Autodesk Fusion 360 part; units mm, degrees
sketch "Sketch1" plane through (0, 0, 0) normal (0, 1, 0) x (1, 0, 0)
  circle A0 centre (0, 0) radius 10.5
  circle A1 centre (0, -0.5) radius 9.25
  line L0 (8, 12) -> (0, 0)
  line L1 (0, 0) -> (-8, 12)
  line L2 (-12, -8) -> (0, 0)
  line L3 (0, 0) -> (12, -8)
  circle A2 centre (0, 0) radius 8
  line L4 (6, 8) -> (6, -7)
  line L5 (-6, 8) -> (-6, -7)
  point P0 (0, -0.5)
  dimension "d1" = 21
  dimension "d2" = 0.5
  dimension "d3" = 18.5
  dimension "d4" = 16
extrude "Extrude1" add sketch "Sketch1" along normal blind 9 contours A0 A1 L0 L3 | A0 A1 L2 L3 | A0 A1 L1 L2 | A1 L0 A2 L4 | A1 L3 A2 L4 | A1 L2 L3 A2 | A1 L1 A2 L5 | A1 L2 A2 L5
extrude "Extrude2" add sketch "Sketch1" against normal blind 20 contours A0 A1 L0 L3 | A0 A1 L1 L2
extrude "Extrude3" add sketch "Sketch1" along normal blind 2 contours L3 A2 L4 | L3 A2 L4 | L2 A2 L5 | L2 A2 L5
chamfer "Chamfer1" distance 1.5 angle 45 1 edges at (8, 2, 0)
chamfer "Chamfer1" distance 1.5 angle 45 1 edges at (-8, 2, 0)
mirror "Mirror1" about plane through (0, 9, 0) normal (0, 1, 0) of bodies 1 merged
Here's how the part is built. I have some questions about the finished solid (model axes, mm). A direction names the side the tool comes from. Coordinates: 2 decimals unless noted, no trailing zeros. Loops run counter-clockwise (first coordinate to the right, second up) from the corner with the lowest first, then second, coordinate; pieces in that order, holes last.
1. Imagine slicing it at B-B, the plane z = 0. Please give me the cut outline in (x, y).
2. Imagine slicing it at A-A, the plane y = 25. Please give me the cut outline in (x, z), and give its area (3 significant figures).
3. Imagine slicing it at C-C, the plane x = -2.75. Please give me the cut outline in (y, z), and give its area (3 significant figures).
4. I need wall thicknesses on L1, parallel to Y at x = -2.5, z = 9; L2, parallel to X at y = 10.5, z = 0; L3, parallel to X at y = -6.5, z = -7. Which ranges of each line are inside material? Lowest first, please.
5. For faces 1 (the flat face through (-4, 18, 7.4)), 2 (the conical face through (-7.1, 15.4, 0.1)), 3 (the cylindrical face through (9.02, -9.86, -1.55)), which set-ups out of +Z, -Z, +X, -X, +Y, -Y let a thin tool reach every point of the face, with its end or its side?
6. If we mould it in two halves opening along X, with no side actions, what happens to faces 4 (the flat face through (9, -20, -3)), 5 (the cylindrical face through (0.375, 8.594, 10.493)), 6 (the cylindrical face through (-8.972, -9.86, -1.751)), 7 (the flat face through (6, 17, 0))? For each: pulls with the +X half, pulls with the -X half, needs draft (parallel to the pull), parting line crosses it, or undercut.
7. Imagine slicing it at D-D, the plane z = -6. Please give me the cut outline in (x, y), and give its area (3 significant figures).
8. For P1, Ø0.6, axis at x = 6.5, z = -0.5, coming from the -Y side; P2, Ø1.1, axis at y = 1.5, z = 2.5, coming from the +X side; P3, Ø1, axis at x = 3.5, y = 0, coming from the +Z side, each with a flat end and sliding along its axis, tell me the tip position at first contact or that it passes through.
Taken from the geometry:
1. outline: (-10.5, -20) - (-9.24, -20) - (-9.24, 0) - (-6, 0) - (-6, 2) - (-6.5, 2) - (-8, 3.5) - (-8, 14.5) - (-6.5, 16) - (-6, 16) - (-6, 18) - (-9.24, 18) - (-9.24, 38) - (-10.5, 38) - close; (6, 0) - (9.24, 0) - (9.24, -20) - (10.5, -20) - (10.5, 38) - (9.24, 38) - (9.24, 18) - (6, 18) - (6, 16) - (6.5, 16) - (8, 14.5) - (8, 3.5) - (6.5, 2) - (6, 2) - close
2. outline: (-8.74, 5.82) arc R10.5 ccw to (-5.82, -8.74) - (-4.9, -7.35) arc R9.25 cw to (-7.92, 5.28) - close; (4.9, -7.35) - (5.82, -8.74) arc R10.5 ccw to (8.74, 5.82) - (7.92, 5.28) arc R9.25 cw to start
2. area: 41.6 mm2
3. outline: (0, 7.51) - (18, 7.51) - (18, 10.13) - (0, 10.13) - close
3. area: 47.2 mm2
4. L1: y = 0 to 18
4. L2: x = -10.5 to -8, 8 to 10.5
4. L3: x = -7.83 to -5.41, 5.41 to 7.83
5. face 1: +Y
5. face 2: none
5. face 3: -Y
6. face 4: needs draft
6. face 5: parting line crosses it
6. face 6: undercut
6. face 7: undercut
7. outline: (-8.62, -20) - (-6.58, -20) - (-6.58, 0) - (-5.29, 0) - (-5.29, 18) - (-6.58, 18) - (-6.58, 38) - (-8.62, 38) - close; (5.29, 0) - (6.58, 0) - (6.58, -20) - (8.62, -20) - (8.62, 38) - (6.58, 38) - (6.58, 18) - (5.29, 18) - close
7. area: 283 mm2
8. P1: stops at y = 0
8. P2: stops at x = 10.32
8. P3: stops at z = 10.06
